Input: part model. Units: mm. Frame: model coordinates. A direction names the side the tool comes from. Coordinates: 2 decimals unless noted, no trailing zeros. Order: outer loops, then holes, each group sorted by start corner. A loop starts at its lowest first (then second) coordinate and runs counter-clockwise, first axis right, second up. Notation, with made-up numbers: M 74.25,76 L 109.25,76 A5 cw 109.25,81 Z; hole C 70.5,85 d9. An arc over 180 degrees is marked long. Answer in a Markdown table with one row per item.
from build123d import *


with BuildPart() as f1:
    # F0 (on Front) → F1 (revolve)
    with BuildSketch(Plane.XZ):
        with BuildLine():
            Line((0, 48.26), (0, 0))
            Line((0, 0), (5.08, 0))
            Line((5.08, 0), (2.8448, 67.275295))
            ThreePointArc((2.8448, 67.275295), (0.835988, 71.802632), (-3.755558, 73.66))
            Line((-3.755558, 73.66), (-6.477, 73.66))
            Line((-6.477, 73.66), (-6.477, 48.26))
            Line((-6.477, 48.26), (0, 48.26))
        make_face()
        Polygon((5.08, 0), (0, 0), (0, -27.94), (6.008297, -27.94), align=None)
    revolve(axis=Axis((-6.477, 0, 60.96), (0, 0, -1)))


solid = f1.part
1) Contact query for flat-ended pins moving along their axis: pin 1 (12 mm diameter, centred on y = 9.5, z = 50, fed in from -X); pin 2 (4 mm diameter, centred on x = -2.5, z = 54.5, fed in from -Y); pin 3 (4 mm diameter, centred on x = -15.5, z = 47, fed in from -Y). Output: stop coordinate, or through.
Resolved:
| item | result |
|---|---|
| pin 1 | stops at x = -15.74 |
| pin 2 | stops at y = -9.55 |
| pin 3 | stops at y = -7.11 |
2) Cut plane A-A, the plane z = 5.5. Output: boundary loops of the cut face in (x, y).
Resolved:
| item | result |
|---|---|
| outline | C -6.48,0 d22.75; hole C -6.48,0 d12.95 |
3) Cut plane C-C, the plane z = 30. Output: boundary loops of the cut face in (x, y), and give its area (3 significant figures).
Resolved:
| item | result |
|---|---|
| outline | C -6.48,0 d21.12; hole C -6.48,0 d12.95 |
| area | 219 mm2 |
4) Mould query, pull axis X, two halves, no side actions, for faces 3 (the face through (-0.5, 2.5, 9.6)), 4 (the face through (-7, 0, 73.66)). Classes: +X half, -X half, draft (parallel to the pull), parting line (faces both ways), or undercut.
Resolved:
| item | result |
|---|---|
| face 3 | undercut |
| face 4 | draft |
5) Reachability of faces 1 (the face through (-12, 5, -27.94)), 2 (the face through (-6, 0, 48.26)) from +Z, -Z, +X, -X, +Y, -Y: full face, straight path, thin tool, end or side. Return the list, or none.
Resolved:
| item | result |
|---|---|
| face 1 | -Z, +X, -X, +Y, -Y |
| face 2 | -Z |
6) Cut plane B-B, the plane z = 63.5. Output: boundary loops of the cut face in (x, y), and give its area (3 significant figures).
Resolved:
| item | result |
|---|---|
| outline | C -6.48,0 d18.89 |
| area | 280 mm2 |
7) Material intervals for probe 1 along X at (y, z) = (0, 0.5); probe 2 along X at (y, z) = (0.5, -21); probe 3 along Y at (x, z) = (-7.75, 9.5), sorted ascending.
Resolved:
| item | result |
|---|---|
| probe 1 | x = -18.02 to -12.95, 0 to 5.06 |
| probe 2 | x = -18.72 to -12.93, -0.02 to 5.77 |
| probe 3 | y = -11.17 to -6.35, 6.35 to 11.17 |
